Verification items for the finished model (mm, model axes). A direction names the side the tool comes from. Coordinates: 2 decimals unless noted, no trailing zeros. Order: outer loops, then holes, each group sorted by start corner. A loop starts at its lowest first (then second) coordinate and runs counter-clockwise, first axis right, second up. Notation, with made-up numbers: M 8.5,10.25 L 42.5,10.25 A9 cw 42.5,16.25 Z; hole C 53,-10 d9. An arc over 180 degrees is marked long. Use one line per item in the form item = value. Start each with the question number.
```python
from build123d import *

# Parameters (mm, degrees)
BOSS_EXTRUDE1_DEPTH      = 35
FILLET1_R                = 2
FILLET2_R                = 2
SKETCH4_W                = 28
SKETCH4_H                = 14
CUT_EXTRUDE2_DEPTH       = 2
FILLET3_R                = 2
FILLET4_R                = 2
F_4_0_4_DIAMETER_HOLE1_D = 4


with BuildPart() as part:
    # Sketch1 → Boss-Extrude1 (new body)
    with BuildSketch(Plane.XY):
        Polygon((-12, 3.174979041), (-12, -12.825020959), (-24, -12.825020959), (-24, -10.825020959), (-14, -10.825020959), (-14, 5.174979041), (14, 5.174979041), (14, -10.825020959), (24, -10.825020959), (24, -12.825020959), (12, -12.825020959), (12, 3.174979041), align=None)
    extrude(amount=-BOSS_EXTRUDE1_DEPTH)

    # Fillet1
    fillet1_edges = [part.edges().sort_by_distance(p)[0] for p in [
        (-14, 5.174979041, -17.5),
    ]]
    fillet(fillet1_edges, radius=FILLET1_R)

    # Fillet2
    fillet2_edges = [part.edges().sort_by_distance(p)[0] for p in [
        (14, 5.174979041, -17.5),
    ]]
    fillet(fillet2_edges, radius=FILLET2_R)

    # Sketch4 → Cut-Extrude2 (cut)
    with BuildSketch(Plane(origin=(0, 5.174979041, 0), x_dir=(1, 0, 0), z_dir=(0, 1, 0))):
        with Locations((0, 7)):
            Rectangle(SKETCH4_W, SKETCH4_H)
    extrude(amount=-CUT_EXTRUDE2_DEPTH, mode=Mode.SUBTRACT)

    # Fillet3
    fillet3_edges = [part.edges().sort_by_distance(p)[0] for p in [
        (12, -12.825020959, -17.5),
    ]]
    fillet(fillet3_edges, radius=FILLET3_R)

    # Fillet4
    fillet4_edges = [part.edges().sort_by_distance(p)[0] for p in [
        (-12, -12.825020959, -17.5),
    ]]
    fillet(fillet4_edges, radius=FILLET4_R)

    # Ø4.0 (4) Diameter Hole1 (through all)
    with Locations(Plane(origin=(0, 5.174979041, 0), x_dir=(1, 0, 0), z_dir=(0, 1, 0))):
        with Locations((-19, 30), (-19, 5), (0, 27), (0, 19), (19, 30), (19, 5)):
            Hole(F_4_0_4_DIAMETER_HOLE1_D / 2)


solid = part.part
```
1. Cross-section at D-D on y = -8.25. Enter the section's corners in (x, z), and give its area (3 significant figures).
2. Cross-section at B-B on z = -5. Enter the section's corners in (x, y).
3. Depth check by flat-ended pin: P1, Ø1, axis at x = 11, y = -6.5, coming from the -Z side; P2, Ø2, axis at x = -5.5, y = 4.5, coming from the +Z side; P3, Ø17, axis at x = 4.5, z = -27.5, coming from the -Y side; P4, Ø7, axis at y = -5, z = -16.5, coming from the -X side. Enter the tip coordinate at first touch or a pass-through.
4. Cross-section at C-C on x = 19. Enter the section's corners in (y, z), and give its area (3 significant figures).
5. Tool access check on faces 1 (the flat face through (-12, -4, -17)), 2 (the flat face through (14, -4, -17)), 3 (the flat face through (0, 4, -14)). Record the directions out of +Z, -Z, +X, -X, +Y, -Y that give a thin tool (end or side, any length) a straight path to the whole face; none if there is none.
6. Material ranges on line 1 along Z through (x, y) = (19, -12.4); line 2 along Z through (x, y) = (0, 3.8); line 3 along X through (y, z) = (1.75, -24), recorded low to high.
7. Cross-section at A-A on z = -27. Enter the section's corners in (x, y).
Final values:
q1.outline = M -14,-35 L -12,-35 L -12,0 L -14,0 Z; M 12,-35 L 14,-35 L 14,0 L 12,0 Z
q1.area = 140 mm2
q2.outline = M -24,-12.83 L -21,-12.83 L -21,-10.83 L -24,-10.83 Z; M -17,-12.83 L -14,-12.83 A2 ccw -12,-10.83 L -12,3.17 L -14,3.17 L -14,-10.83 L -17,-10.83 Z; M 12,-10.83 A2 ccw 14,-12.83 L 17,-12.83 L 17,-10.83 L 14,-10.83 L 14,3.17 L 12,3.17 Z; M 21,-12.83 L 24,-12.83 L 24,-10.83 L 21,-10.83 Z
q3.P1 = through
q3.P2 = -14
q3.P3 = -12.56
q3.P4 = -14
q4.outline = M -12.83,-35 L -10.83,-35 L -10.83,-32 L -12.83,-32 Z; M -12.83,-28 L -10.83,-28 L -10.83,-7 L -12.83,-7 Z; M -12.83,-3 L -10.83,-3 L -10.83,0 L -12.83,0 Z
q4.area = 54.0 mm2
q5.face_1 = +Z, -Z, -Y
q5.face_2 = +Z, -Z, +X, +Y
q5.face_3 = +Z, +X, -X, +Y
q6.line_1 = -35 to -32, -28 to -7, -3 to 0
q6.line_2 = -35 to -29, -25 to -21, -17 to -14
q6.line_3 = -14 to -12, 12 to 14
q7.outline = M -24,-12.83 L -14,-12.83 A2 ccw -12,-10.83 L -12,3.17 L -2,3.17 L -2,5.17 L -12,5.17 A2 ccw -14,3.17 L -14,-10.83 L -24,-10.83 Z; M 2,3.17 L 12,3.17 L 12,-10.83 A2 ccw 14,-12.83 L 24,-12.83 L 24,-10.83 L 14,-10.83 L 14,3.17 A2 ccw 12,5.17 L 2,5.17 Z
